from build123d import *

# Parameters (mm, degrees)
F1_DEPTH = 40
F0_W     = 20
F0_H     = 20
F2_DEPTH = 40
F4_DEPTH = 20


with BuildPart() as f1:
    # F0 (on Front) → F1 (new body)
    with BuildSketch(Plane.XZ):
        Polygon((0, 20), (0, 0), (50, 0), (50, 10), (20, 20), align=None)
    extrude(amount=F1_DEPTH)

    # F0 (on Front) → F2 (join)
    with BuildSketch(Plane.XZ):
        with Locations((10, 30)):
            Rectangle(F0_W, F0_H)
    extrude(amount=F2_DEPTH)

    # F3 (on face) → F4 (cut)
    with BuildSketch(Plane.YZ.offset(20)):
        Polygon((-40, 20), (-20, 40), (-40, 40), align=None)
    extrude(amount=-F4_DEPTH, mode=Mode.SUBTRACT)


solid = f1.part
The model under review builds one solid part; all positions refer to its coordinate system, in mm. A direction names the side the tool comes from. Coordinates: 2 decimals unless noted, no trailing zeros. Write each loop counter-clockwise with the first axis right and the second up, starting at its lowest first coordinate (ties: lowest second). Pieces come first, ordered by that corner, then holes. Notation, with made-up numbers: (-3, -23) - (53, -23) arc R29 cw to (53, -2) - close; hole circle Ø7 at (58.25, -35.75). An arc over 180 degrees is marked (long way). Answer as a JSON object with one key per item and string values. Group by question number.
1. Clearance check with flat-ended pins moving along their axes: pin 1 Ø1.5 at (y, z) = (-10, 22) entering from -X; pin 2 Ø6 at (y, z) = (-15, 26) entering from +X; pin 3 Ø4 at (x, z) = (23.5, 32.5) entering from -Y. State where each tip first meets the part, or that it passes through.
2. Add section B-B (y = -23.5). Give the boundary of the cut face in (x, z), plus the area to 3 significant figures.
3. Machinability: for faces 1 (the face through (25, -40, 8)), 2 (the face through (20, -15, 30)), which of the approach directions +Z, -Z, +X, -X, +Y, -Y give a long, thin tool a straight path to every point of the face, cutting with its end or side? Answer none if there is none.
4. To check wall thickness, follow probe 1 along X at (y, z) = (-33, 26); probe 2 along Z at (x, y) = (30, -27.5); probe 3 along Y at (x, z) = (6, 21.5). State the ranges of each line that lie inside material, in increasing order.
5. Add section D-D (y = -34). Give the boundary of the cut face in (x, z).
6. Add section C-C (z = 26). Give the boundary of the cut face in (x, y).
7. Add section A-A (x = 8). Give the boundary of the cut face in (y, z).
Findings:
{
 "1": {"pin 1": "x = 0", "pin 2": "x = 20", "pin 3": "through"},
 "2": {"outline": "(0, 0) - (50, 0) - (50, 10) - (20, 20) - (20, 36.5) - (0, 36.5) - close", "area": "1,180 mm²"},
 "3": {"face 1": "+Z, -Z, +X, -X, -Y", "face 2": "+Z, +X, +Y, -Y"},
 "4": {"probe 1": "0 to 20", "probe 2": "0 to 16.67", "probe 3": "-38.5 to 0"},
 "5": {"outline": "(0, 0) - (50, 0) - (50, 10) - (20, 20) - (20, 26) - (0, 26) - close"},
 "6": {"outline": "(0, -34) - (20, -34) - (20, 0) - (0, 0) - close"},
 "7": {"outline": "(-40, 0) - (0, 0) - (0, 40) - (-20, 40) - (-40, 20) - close"}
}
